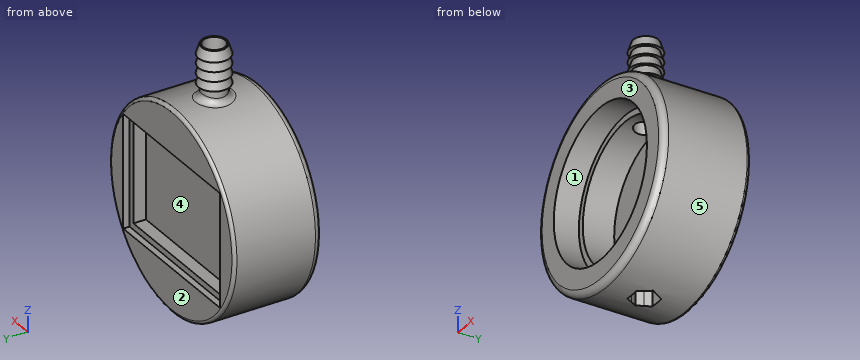
```python
from build123d import *

# Parameters (mm, degrees)
F0_R           = 50.8
F1_DEPTH       = 44.45
F2_R           = 34.925
F3_DEPTH       = 28.575
F4_R           = 38.1
F5_DEPTH       = 12.7
F8_R           = 3.175
F9_R           = 1.5875
F12_DEPTH      = 25.4
F13_R          = 5.55625
F14_DEPTH      = 17.4625
F15_R          = 6.35
F15_R_2        = 5.55625
F16_DEPTH      = 26.67
F20_R          = 3.175
F22_W          = 73.025
F22_H          = 50.8
F23_DEPTH      = 9.525
F22_W_2        = 79.375
F22_H_2        = 57.15
F24_DEPTH      = 3.175
F24_DEPTH_BACK = 25.4


with BuildPart() as f1:
    # F0 (on Front) → F1 (new body)
    with BuildSketch(Plane.XZ):
        Circle(F0_R)
    extrude(amount=-F1_DEPTH)

    # F2 (on Front) → F3 (cut)
    with BuildSketch(Plane.XZ):
        Circle(F2_R)
    extrude(amount=-F3_DEPTH, mode=Mode.SUBTRACT)

    # F4 (on Front) → F5 (cut)
    with BuildSketch(Plane.XZ):
        Circle(F4_R)
    extrude(amount=-F5_DEPTH, mode=Mode.SUBTRACT)

    # F8
    f8_edges = [f1.edges().sort_by_distance(p)[0] for p in [
        (-50.8, 0, 0),
    ]]
    fillet(f8_edges, radius=F8_R)

    # F9
    f9_edges = [f1.edges().sort_by_distance(p)[0] for p in [
        (-50.8, 44.45, 0),
    ]]
    fillet(f9_edges, radius=F9_R)

    # F11 (on offset) → F12 (cut)
    with BuildSketch(Plane.XY.offset(-50.8)):
        with BuildLine():
            ThreePointArc((5.4992612052, 19.0499998116), (6.1336289688, 20.5814989585), (6.35, 22.225))
            ThreePointArc((6.35, 22.225), (6.1336290298, 23.8685008137), (5.4992614411, 25.3999997799))
            ThreePointArc((5.4992614411, 25.3999997799), (3.17500011, 27.7242612505), (0, 28.575))
            ThreePointArc((0, 28.575), (-3.1749999058, 27.7242613684), (-5.4992612052, 25.4000001884))
            ThreePointArc((-5.4992612052, 25.4000001884), (-6.35, 22.2249999281), (-5.4992611333, 19.049999687))
            ThreePointArc((-5.4992611333, 19.049999687), (-3.1749998435, 16.7257385956), (0, 15.875))
            ThreePointArc((0, 15.875), (3.1749999058, 16.7257386316), (5.4992612052, 19.0499998116))
        make_face()
        with BuildLine():
            ThreePointArc((0, 28.575), (3.17500011, 27.7242612505), (5.4992614411, 25.3999997799))
            Line((5.4992614411, 25.3999997799), (3.6661742094, 28.575))
            Line((3.6661742094, 28.575), (0, 28.575))
        make_face()
        with BuildLine():
            ThreePointArc((-5.4992612052, 25.4000001884), (-3.1749999058, 27.7242613684), (0, 28.575))
            Line((0, 28.575), (-3.6661742094, 28.575))
            Line((-3.6661742094, 28.575), (-5.4992612052, 25.4000001884))
        make_face()
        with BuildLine():
            ThreePointArc((-5.4992611333, 19.049999687), (-6.35, 22.2249999281), (-5.4992612052, 25.4000001884))
            Line((-5.4992612052, 25.4000001884), (-7.3323484187, 22.225))
            Line((-7.3323484187, 22.225), (-5.4992611333, 19.049999687))
        make_face()
        with BuildLine():
            Line((-3.6661742094, 15.875), (0, 15.875))
            ThreePointArc((0, 15.875), (-3.1749998435, 16.7257385956), (-5.4992611333, 19.049999687))
            Line((-5.4992611333, 19.049999687), (-3.6661742094, 15.875))
        make_face()
        with BuildLine():
            Line((3.6661742094, 15.875), (5.4992612052, 19.0499998116))
            ThreePointArc((5.4992612052, 19.0499998116), (3.1749999058, 16.7257386316), (0, 15.875))
            Line((0, 15.875), (3.6661742094, 15.875))
        make_face()
        with BuildLine():
            ThreePointArc((5.4992614411, 25.3999997799), (6.1336290298, 23.8685008137), (6.35, 22.225))
            ThreePointArc((6.35, 22.225), (6.1336289688, 20.5814989585), (5.4992612052, 19.0499998116))
            Line((5.4992612052, 19.0499998116), (7.3323484187, 22.225))
            Line((7.3323484187, 22.225), (5.4992614411, 25.3999997799))
        make_face()
    extrude(amount=F12_DEPTH, mode=Mode.SUBTRACT)

    # F13 (on offset) → F14 (cut)
    with BuildSketch(Plane.XY.offset(50.8)):
        with Locations((0, 23.01875)):
            Circle(F13_R)
    extrude(amount=-F14_DEPTH, mode=Mode.SUBTRACT)


with BuildPart() as f16:
    # F15 (on offset) → F16 (new body)
    with BuildSketch(Plane.XY.offset(50.8)):
        with Locations((0, 23.01875)):
            Circle(F15_R)
        with Locations((0, 23.01875)):
            Circle(F15_R_2, mode=Mode.SUBTRACT)
    extrude(amount=F16_DEPTH)


with BuildPart() as f16_1:
    # F18: moved
    add(f16.part.moved(Location((0, 0, -0.508))))

    # F19: union F1
    add(f1.part)

    # F20
    f20_edges = [f16_1.edges().sort_by_distance(p)[0] for p in [
        (-6.35, 23.01875, 50.401562),
    ]]
    fillet(f20_edges, radius=F20_R)

    # F17 (on Right) → F21 (revolve)
    with BuildSketch(Plane.YZ):
        Polygon((16.66875, 67.2536837804), (16.66875, 72.0792659992), (15.08125, 67.2536837804), align=None)
        Polygon((16.66875, 62.4281015617), (16.66875, 67.2536837804), (15.08125, 62.4281015617), align=None)
        Polygon((16.66875, 57.6025193429), (16.66875, 62.4281015617), (15.08125, 57.6025193429), align=None)
        Polygon((16.66875, 72.0792659992), (16.66875, 76.904848218), (15.08125, 72.0792659992), align=None)
    revolve(axis=Axis((0, 23.01875, 64.9531239529), (0, 0, -1)))

    # F22 (on offset) → F23 (cut)
    with BuildSketch(Plane.XZ.offset(-44.45)):
        Rectangle(F22_W, F22_H)
    extrude(amount=F23_DEPTH, mode=Mode.SUBTRACT)

    # F22 (on offset) → F24 (cut, two sides)
    with BuildSketch(Plane.XZ.offset(-44.45)) as f24_sk:
        Rectangle(F22_W_2, F22_H_2)
        Rectangle(F22_W, F22_H, mode=Mode.SUBTRACT)
    extrude(amount=F24_DEPTH, mode=Mode.SUBTRACT)
    extrude(f24_sk.sketch, amount=-F24_DEPTH_BACK, mode=Mode.SUBTRACT)


solid = f16_1.part
```
Here's how the part is built. I have some questions about the finished solid (model axes, mm). Face numbers are marked on the shaded views. A direction names the side the tool comes from. Coordinates: 2 decimals unless noted, no trailing zeros. Order: outer loops, then holes, each group sorted by start corner. A loop starts at its lowest first (then second) coordinate and runs counter-clockwise, first axis right, second up. Notation, with made-up numbers: (-29, -5) -> (17, -5) arc R30 ccw to (17, 28) -> close; hole circle Ø6 at (44, -4.75). An arc over 180 degrees is marked (long way). Return JSON: item names as keys, results as strings.
1) Thinking about a two-plate mould opening in Z: for the marked faces 3, 4 and 5, which applies, +Z half, -Z half, draft (parallel to the pull), parting line (faces both ways), or undercut?
Conclusion:
{"face 3": "draft", "face 4": "undercut", "face 5": "parting line"}
2) I'm going to push flat-ended pins straight in: P1, Ø3.5, axis at x = -18, y = 42.5, coming from the -Z side; P2, Ø5, axis at x = 13.5, y = 38, coming from the -Z side; P3, Ø1.9, axis at y = 39.5, z = 7, coming from the +X side; P4, Ø5, axis at x = 2, y = 24, coming from the -Z side. Where does each tip first touch, or does it pass through?
Conclusion:
{"P1": "stops at z = -48.13", "P2": "stops at z = -49.59", "P3": "stops at x = 50.44", "P4": "passes through"}
3) If I drill on probe 1 along X at (y, z) = (22.5, -0.5); probe 2 along X at (y, z) = (20.5, -5.5); probe 3 along Y at (x, z) = (0, 56) (1 decimal), over which ranges is the centre line in solid material (lowest first)?
Conclusion:
{"probe 1": "x = -50.8 to -34.92, 34.92 to 50.8", "probe 2": "x = -50.5 to -34.49, 34.49 to 50.5", "probe 3": "y = 16.7 to 17.5, 28.6 to 29.4"}
4) On a 3-axis mill with a long thin cutter (end or side, diameter ignored), from which of +Z, -Z, +X, -X, +Y, -Y can I reach the whole of each face in a straight line? I mean the marked faces 1 and 2. Say none if no direction works.
Conclusion:
{"face 1": "-Y", "face 2": "+Z, -Z, +X, -X, +Y"}
5) If we section it at A-A on y = 38.5: List the corners of the cut face in (x, z) for me.
Conclusion:
{"outline": "circle Ø101.6 at (0, 0); hole (-36.51, -25.4) -> (36.51, -25.4) -> (36.51, 25.4) -> (-36.51, 25.4) -> close"}
6) If we section it at C-C on y = 5: List the corners of the cut face in (x, z) for me, plus the area to 3 significant figures.
Conclusion:
{"outline": "circle Ø101.6 at (0, 0); hole circle Ø76.2 at (0, 0)", "area": "3,550 mm²"}
